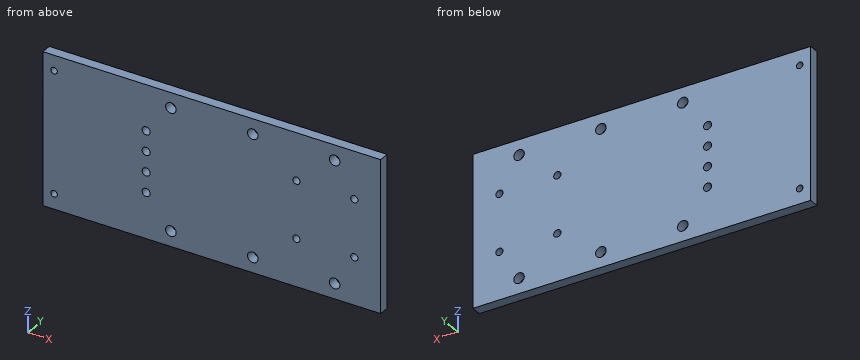
from build123d import *

# Parameters (mm, degrees)
SKETCH1_W           = 209.55
SKETCH1_H           = 95.25
BOSS_EXTRUDE1_DEPTH = 6.35
SKETCH2_R           = 2.0193
CUT_EXTRUDE1_DEPTH  = 7.35
SKETCH3_R           = 2.4892
CUT_EXTRUDE2_DEPTH  = 7.35
SKETCH4_R           = 2.2479
CUT_EXTRUDE3_DEPTH  = 7.35
SKETCH5_R           = 3.2639
CUT_EXTRUDE4_DEPTH  = 7.35


with BuildPart() as part:
    # Sketch1 → Boss-Extrude1 (new body)
    with BuildSketch(Plane(origin=(0, 0, 0), x_dir=(1, 0, 0), z_dir=(0, 1, 0))):
        Rectangle(SKETCH1_W, SKETCH1_H)
    extrude(amount=BOSS_EXTRUDE1_DEPTH)

    # Sketch2 → Cut-Extrude1 (cut, through all)
    with BuildSketch(Plane(origin=(0, 6.35, 0), x_dir=(1, 0, 0), z_dir=(0, 1, 0))):
        with Locations((-97.917, -38.1)):
            Circle(SKETCH2_R)
    cut_extrude1 = extrude(amount=-CUT_EXTRUDE1_DEPTH, mode=Mode.SUBTRACT)

    # Mirror1: Cut-Extrude1 across plane
    add(cut_extrude1.mirror(Plane.XY), mode=Mode.SUBTRACT)

    # Sketch3 → Cut-Extrude2 (cut, through all)
    with BuildSketch(Plane(origin=(0, 6.35, 0), x_dir=(1, 0, 0), z_dir=(0, 1, 0))):
        with Locations((-40.767, -6.35)):
            Circle(SKETCH3_R)
        with Locations((-40.767, -19.05)):
            Circle(SKETCH3_R)
    cut_extrude2 = extrude(amount=-CUT_EXTRUDE2_DEPTH, mode=Mode.SUBTRACT)

    # Mirror2: Cut-Extrude2 across plane
    add(cut_extrude2.mirror(Plane.XY), mode=Mode.SUBTRACT)

    # Sketch4 → Cut-Extrude3 (cut, through all)
    with BuildSketch(Plane(origin=(0, 6.35, 0), x_dir=(1, 0, 0), z_dir=(0, 1, 0))):
        with Locations((52.47132, 17.96034)):
            Circle(SKETCH4_R)
        with Locations((88.392, 17.96034)):
            Circle(SKETCH4_R)
        with Locations((88.392, -17.96034)):
            Circle(SKETCH4_R)
        with Locations((52.47132, -17.96034)):
            Circle(SKETCH4_R)
    extrude(amount=-CUT_EXTRUDE3_DEPTH, mode=Mode.SUBTRACT)

    # Sketch5 → Cut-Extrude4 (cut, through all)
    with BuildSketch(Plane(origin=(0, 6.35, 0), x_dir=(1, 0, 0), z_dir=(0, 1, 0))):
        with Locations((-25.4, 38.1)):
            Circle(SKETCH5_R)
        with Locations((25.4, 38.1)):
            Circle(SKETCH5_R)
        with Locations((76.2, 38.1)):
            Circle(SKETCH5_R)
    cut_extrude4 = extrude(amount=-CUT_EXTRUDE4_DEPTH, mode=Mode.SUBTRACT)

    # Mirror3: Cut-Extrude4 across plane
    add(cut_extrude4.mirror(Plane.XY), mode=Mode.SUBTRACT)


solid = part.part
Model file for the job. Use its own axes, mm. Coordinates: 2 decimals unless noted, no trailing zeros. Write each loop counter-clockwise with the first axis right and the second up, starting at its lowest first coordinate (ties: lowest second). Pieces come first, ordered by that corner, then holes. Notation, with made-up numbers: (40.25, 28.25) -> (64.25, 28.25) arc R16 cw to (64.25, 41.25) -> close; hole circle Ø3 at (35.25, 23.5). An arc over 180 degrees is marked (long way). One line per item, written item: value. Start each with the question number.
1) Probe probe 1 along X at (y, z) = (5, -38.1) (3 decimals); probe 2 along X at (y, z) = (5.5, 19) (3 decimals); probe 3 along X at (y, z) = (3, -19.05) (3 decimals). List the from-to ranges inside material, lowest first.
2) Slice it at C-C on z = -38.1. Write the cut outline in (x, y) (3 decimals), then the cut area to 3 significant figures.
3) Slice it at B-B on x = -25.4. Write the cut outline in (y, z) (3 decimals).
4) Slice it at A-A on z = 6.35. Write the cut outline in (x, y) (3 decimals).
5) Slice it at D-D on y = 1.5. Count the separate pieces of the cut face and the enclosed holes in it, then the cut area to 3 significant figures.
Answers follow:
1. probe 1: -104.775 to -99.936, -95.898 to -28.664, -22.136 to 22.136, 28.664 to 72.936, 79.464 to 104.775
1. probe 2: -104.775 to -43.256, -38.278 to 50.478, 54.464 to 86.399, 90.385 to 104.775
1. probe 3: -104.775 to -43.256, -38.278 to 50.505, 54.437 to 86.426, 90.358 to 104.775
2. outline: (-104.775, 0) -> (-99.936, 0) -> (-99.936, 6.35) -> (-104.775, 6.35) -> close; (-95.898, 0) -> (-28.664, 0) -> (-28.664, 6.35) -> (-95.898, 6.35) -> close; (-22.136, 0) -> (22.136, 0) -> (22.136, 6.35) -> (-22.136, 6.35) -> close; (28.664, 0) -> (72.936, 0) -> (72.936, 6.35) -> (28.664, 6.35) -> close; (79.464, 0) -> (104.775, 0) -> (104.775, 6.35) -> (79.464, 6.35) -> close
2. area: 1,180 mm2
3. outline: (0, -47.625) -> (6.35, -47.625) -> (6.35, -41.364) -> (0, -41.364) -> close; (0, -34.836) -> (6.35, -34.836) -> (6.35, 34.836) -> (0, 34.836) -> close; (0, 41.364) -> (6.35, 41.364) -> (6.35, 47.625) -> (0, 47.625) -> close
4. outline: (-104.775, 0) -> (-43.256, 0) -> (-43.256, 6.35) -> (-104.775, 6.35) -> close; (-38.278, 0) -> (104.775, 0) -> (104.775, 6.35) -> (-38.278, 6.35) -> close
5. separate pieces: 1
5. enclosed holes: 16
5. area: 19,600 mm2
